Could you check a few things on this model? Use its own coordinates, in mm. A direction names the side the tool comes from. Give positions to 0.01 mm unless a question says otherwise; leave off trailing zeros. Write each loop counter-clockwise with the first axis right and the second up, starting at its lowest first coordinate (ties: lowest second). Pieces come first, ordered by that corner, then holes. Notation, with made-up numbers: (-29.5, 88.25) -> (-2.5, 88.25) arc R9 ccw to (-2.5, 96.25) -> close; hole circle Ø10 at (58, 17.25). An arc over 180 degrees is marked (long way). Write item = value, one per line. Start each with the question number.
```python
from build123d import *

# Parameters (mm, degrees)
F1_DEPTH = 11
F3_W     = 3
F3_H     = 20
F3_W_2   = 3.4
F3_H_2   = 10.2
F4_DEPTH = 25
F5_R     = 1.5
F6_DEPTH = 25
F5_R_2   = 2.5
F7_DEPTH = 8
F8_SIZE  = 1.49999
F9_SIZE  = 1.49999


# Not quite as in the source:
# - a fillet or chamfer is up to 0.001 mm smaller than in the source, because OpenCascade refuses the exact size


with BuildPart() as f1:
    # F0 (on Front) → F1 (new body)
    with BuildSketch(Plane.XZ):
        Polygon((-4, 0), (0, 0), (0, 9.8), (-1.7, 9.8), (-1.7, 22.5), (-4, 22.5), align=None)
    extrude(amount=F1_DEPTH)

    # F2: F1 across face


with BuildPart() as f1_1:
    add(f1.part)
    add(f1.part.mirror(Plane(origin=(0, -5.5, 4.9), x_dir=(0, 1, 0), z_dir=(1, 0, 0))))

    # F3 (on face) → F4 (join)
    with BuildSketch(Plane.XZ.offset(11)):
        with Locations((5.5, 10)):
            Rectangle(F3_W, F3_H)
        with Locations((0, 14.9)):
            Rectangle(F3_W_2, F3_H_2)
        Polygon((-4, 0), (0, 0), (4, 0), (4, 20), (1.7, 20), (1.7, 9.8), (-1.7, 9.8), (-1.7, 20), (-4, 20), align=None)
        with Locations((-5.5, 10)):
            Rectangle(F3_W, F3_H)
    extrude(amount=F4_DEPTH)

    # F5 (on face) → F6 (cut)
    with BuildSketch(Plane.YZ.offset(4)):
        with Locations((-4, 16)):
            Circle(F5_R)
    extrude(amount=-F6_DEPTH, mode=Mode.SUBTRACT)

    # F5 (on face) → F7 (join, through all)
    with BuildSketch(Plane.YZ.offset(4)):
        with Locations((-4, 16)):
            Circle(F5_R_2)
        with Locations((-4, 16)):
            Circle(F5_R, mode=Mode.SUBTRACT)
    extrude(amount=-F7_DEPTH)

    # F8 (size 1.5 in the source; OpenCascade refuses exactly that, so slightly less here)
    f8_edges = [f1_1.edges().sort_by_distance(p)[0] for p in [
        (-1.7, -6.5, 16),
    ]]
    chamfer(f8_edges, length=F8_SIZE)

    # F9 (size 1.5 in the source; OpenCascade refuses exactly that, so slightly less here)
    f9_edges = [f1_1.edges().sort_by_distance(p)[0] for p in [
        (1.7, -6.5, 16),
    ]]
    chamfer(f9_edges, length=F9_SIZE)


solid = f1_1.part
```
(1) If I drill on line 1 along Z through (x, y) = (-2, -4); line 2 along Z through (x, y) = (-1, -3); line 3 along Z through (x, y) = (0.75, -4), over which ranges is the centre line in solid material (lowest first)? Write a range as from..to.
(2) Imagine slicing it at B-B (z = 16). State how many separate pieces and enclosed holes the cut face has, then the cut area to 3 significant figures.
(3) On a 3-axis mill with a long thin cutter (end or side, diameter ignored), from which of +Z, -Z, +X, -X, +Y, -Y can I reach the whole of each face in a straight line? I mean faces 1 (the flat face through (0, -11, 15)), 2 (the flat face through (4, -5, 11)), 3 (the flat face through (0, -23, 20)), 4 (the flat face through (7, -23, 10)), 5 (the flat face through (-1.7, -7.9, 17.5)). Say none if no direction works.
(4) Imagine slicing it at D-D (x = -3.5). Please give me the cut outline in (y, z).
(5) Imagine slicing it at C-C (y = -4). Please give me the cut outline in (x, z).
(6) We'd pull the mould along X, two halves only. Please class faces 6 (the flat face through (-3, -5, 22.5)), 7 (the flat face through (-4, -5, 11)), 8 (the cylindrical face through (0, -1.69, 15.04)), 9 (the flat face through (0, -5, 9.8)): released by +X, released by -X, zero draft, split by the parting line, or undercut.
(7) Imagine slicing it at A-A (x = -1.25). Please give me the cut outline in (y, z).
(8) I'm going to push flat-ended pins straight in: pin 1 (1.8 mm diameter, centred on x = 3, z = 21.5, fed in from -Y); pin 2 (1.5 mm diameter, centred on x = -5.5, z = 11.5, fed in from +Y); pin 3 (2 mm diameter, centred on y = -6, z = 17.5, fed in from -X). Where does each tip first touch, or does it pass through?
Answers below:
q1.line_1 = 0..14.5, 17.5..22.5
q1.line_2 = 0..9.8, 12.86..14.88, 17.12..19.14
q1.line_3 = 0..9.8, 12.95..14.5, 17.5..19.05
q2.separate_pieces = 2
q2.enclosed_holes = 1
q2.area = 398 mm^2
q3.face_1 = +Z
q3.face_2 = +Z, -Z, +X, +Y
q3.face_3 = +Z, +X, -X, -Y
q3.face_4 = +Z, -Z, +X, +Y, -Y
q3.face_5 = none
q4.outline = (-36, 0) -> (0, 0) -> (0, 22.5) -> (-11, 22.5) -> (-11, 20) -> (-36, 20) -> close; hole circle Ø3 at (-4, 16)
q5.outline = (-4, 0) -> (4, 0) -> (4, 14.5) -> (-4, 14.5) -> close; (-4, 17.5) -> (4, 17.5) -> (4, 22.5) -> (1.7, 22.5) -> (1.7, 20) -> (0.2, 18.5) -> (-0.2, 18.5) -> (-1.7, 20) -> (-1.7, 22.5) -> (-4, 22.5) -> close; hole (-1.7, 9.8) -> (1.7, 9.8) -> (1.7, 12) -> (0.2, 13.5) -> (-0.2, 13.5) -> (-1.7, 12) -> close
q6.face_6 = zero draft
q6.face_7 = released by -X
q6.face_8 = undercut
q6.face_9 = undercut
q7.outline = (-36, 0) -> (0, 0) -> (0, 9.8) -> (-11, 9.8) -> (-11, 20) -> (-36, 20) -> close; circle Ø7.1 at (-4, 16); hole circle Ø3 at (-4, 16)
q8.pin_1 = -11
q8.pin_2 = -11
q8.pin_3 = -4
